Work out the finished part from the listing and answer in its coordinate system (mm). A direction names the side the tool comes from. Give positions to 0.01 mm unless a question says otherwise; leave off trailing zeros. Loops run counter-clockwise (first coordinate to the right, second up) from the corner with the lowest first, then second, coordinate; pieces in that order, holes last. Notation, with made-up numbers: M 18.25,34 L 22.25,34 A35 ccw 22.25,70 Z; hole C -39,-37 d10. An arc over 180 degrees is marked long. Use a Markdown table: item, result.
```python
from build123d import *

# Parameters (mm, degrees)
SKETCH1_W                 = 188.214
SKETCH1_H                 = 78.74
BOSS_EXTRUDE1_DEPTH       = 0.508
SKETCH1_3_W               = 188.214
SKETCH1_3_H               = 8.255
SKETCH1_3_H_2             = 78.74
SKETCH1_3_W_2             = 183.134
SKETCH1_3_H_3             = 73.66
BOSS_EXTRUDE2_DEPTH       = 27
BOSS_EXTRUDE3_START       = 21.59
BOSS_EXTRUDE3_DEPTH       = 32.5
SKETCH1_4_W               = 188.214
SKETCH1_4_H               = 8.255
BOSS_EXTRUDE4_DEPTH       = 0.508
F_4_40_TAPPED_HOLE2_D     = 2.2606
F_4_40_TAPPED_HOLE2_DEPTH = 7.62
F_4_40_TAPPED_HOLE2_TIP   = 0.679152758
SKETCH11_W                = 114.554
SKETCH11_H                = 8.255
SKETCH11_W_2              = 26.67
CUT_EXTRUDE1_DEPTH        = 28.508


with BuildPart() as part:
    # Sketch1 → Boss-Extrude1 (new body)
    with BuildSketch(Plane(origin=(0, 0, 0), x_dir=(1, 0, 0), z_dir=(0, 1, 0))):
        with Locations((94.107, -39.37)):
            Rectangle(SKETCH1_W, SKETCH1_H)
    extrude(amount=-BOSS_EXTRUDE1_DEPTH)

    # Sketch1<3> → Boss-Extrude2 (add)
    with BuildSketch(Plane(origin=(0, 0, 0), x_dir=(1, 0, 0), z_dir=(0, 1, 0))):
        with Locations((94.107, 4.1275)):
            Rectangle(SKETCH1_3_W, SKETCH1_3_H)
        with Locations((94.107, -82.8675)):
            Rectangle(SKETCH1_3_W, SKETCH1_3_H)
        with Locations((94.107, -39.37)):
            Rectangle(SKETCH1_3_W, SKETCH1_3_H_2)
        with Locations((94.107, -39.37)):
            Rectangle(SKETCH1_3_W_2, SKETCH1_3_H_3, mode=Mode.SUBTRACT)
    extrude(amount=BOSS_EXTRUDE2_DEPTH)

    # Sketch5 → Boss-Extrude3 (add)
    with BuildSketch(Plane.XY.offset(2.54).offset(BOSS_EXTRUDE3_START)):
        with BuildLine():
            Line((29.54, 7), (27.54, 7))
            ThreePointArc((27.54, 7), (23.600043647, 1.985651932), (17.54, 0))
            Line((17.54, 0), (39.54, 0))
            ThreePointArc((39.54, 0), (33.479956353, 1.985651932), (29.54, 7))
        make_face()
        with BuildLine():
            Line((55.4988, 7), (53.4988, 7))
            ThreePointArc((53.4988, 7), (49.558843647, 1.985651932), (43.4988, 0))
            Line((43.4988, 0), (65.4988, 0))
            ThreePointArc((65.4988, 0), (59.438756353, 1.985651932), (55.4988, 7))
        make_face()
        with BuildLine():
            Line((81.4576, 7), (79.4576, 7))
            ThreePointArc((79.4576, 7), (75.517643647, 1.985651932), (69.4576, 0))
            Line((69.4576, 0), (91.4576, 0))
            ThreePointArc((91.4576, 0), (85.397556353, 1.985651932), (81.4576, 7))
        make_face()
        with BuildLine():
            Line((107.4164, 7), (105.4164, 7))
            ThreePointArc((105.4164, 7), (101.476443647, 1.985651932), (95.4164, 0))
            Line((95.4164, 0), (117.4164, 0))
            ThreePointArc((117.4164, 0), (111.356356353, 1.985651932), (107.4164, 7))
        make_face()
        with BuildLine():
            Line((133.3752, 7), (131.3752, 7))
            ThreePointArc((131.3752, 7), (127.435243647, 1.985651932), (121.3752, 0))
            Line((121.3752, 0), (143.3752, 0))
            ThreePointArc((143.3752, 0), (137.315156353, 1.985651932), (133.3752, 7))
        make_face()
        with BuildLine():
            Line((159.334, 7), (157.334, 7))
            ThreePointArc((157.334, 7), (153.394043647, 1.985651932), (147.334, 0))
            Line((147.334, 0), (169.334, 0))
            ThreePointArc((169.334, 0), (163.273956353, 1.985651932), (159.334, 7))
        make_face()
    extrude(amount=BOSS_EXTRUDE3_DEPTH)

    # Sketch1<4> → Boss-Extrude4 (add)
    with BuildSketch(Plane(origin=(0, 0, 0), x_dir=(1, 0, 0), z_dir=(0, 1, 0))):
        with Locations((94.107, 4.1275)):
            Rectangle(SKETCH1_4_W, SKETCH1_4_H)
        with Locations((94.107, -82.8675)):
            Rectangle(SKETCH1_4_W, SKETCH1_4_H)
    extrude(amount=-BOSS_EXTRUDE4_DEPTH)

    # #4-40 Tapped Hole2
    with Locations(Plane(origin=(0, 27, 0), x_dir=(-1, 0, 0), z_dir=(0, 1, 0))):
        with Locations((-31.75, 0), (-156.464, 0), (-31.75, 78.74), (-156.464, 78.74)):
            Hole(F_4_40_TAPPED_HOLE2_D / 2, depth=F_4_40_TAPPED_HOLE2_DEPTH)
            with Locations((0, 0, -(F_4_40_TAPPED_HOLE2_DEPTH + F_4_40_TAPPED_HOLE2_TIP / 2))):  # 118° drill point
                Cone(0, F_4_40_TAPPED_HOLE2_D / 2, F_4_40_TAPPED_HOLE2_TIP, mode=Mode.SUBTRACT)

    # Sketch11 → Cut-Extrude1 (cut, through all)
    with BuildSketch(Plane(origin=(0, 27, 0), x_dir=(1, 0, 0), z_dir=(0, 1, 0))):
        with Locations((94.107, 4.1275)):
            Rectangle(SKETCH11_W, SKETCH11_H)
        with Locations((94.107, -82.8675)):
            Rectangle(SKETCH11_W, SKETCH11_H)
        with Locations((13.335, 4.1275)):
            Rectangle(SKETCH11_W_2, SKETCH11_H)
        with Locations((174.879, 4.1275)):
            Rectangle(SKETCH11_W_2, SKETCH11_H)
        with Locations((174.879, -82.8675)):
            Rectangle(SKETCH11_W_2, SKETCH11_H)
        with Locations((13.335, -82.8675)):
            Rectangle(SKETCH11_W_2, SKETCH11_H)
    extrude(amount=-CUT_EXTRUDE1_DEPTH, mode=Mode.SUBTRACT)


solid = part.part
```
(1) A cutting plane is placed at A-A (y = 12.5). Write down the section's boundary in (x, z) (3 decimals), and give its area (3 significant figures).
Entries:
| item | result |
|---|---|
| outline | M 0,0 L 26.67,0 L 26.67,-8.255 L 36.83,-8.255 L 36.83,0 L 151.384,0 L 151.384,-8.255 L 161.544,-8.255 L 161.544,0 L 188.214,0 L 188.214,78.74 L 161.544,78.74 L 161.544,86.995 L 151.384,86.995 L 151.384,78.74 L 36.83,78.74 L 36.83,86.995 L 26.67,86.995 L 26.67,78.74 L 0,78.74 Z; hole M 2.54,2.54 L 185.674,2.54 L 185.674,76.2 L 2.54,76.2 Z |
| area | 1,670 mm² |
(2) Given P1, Ø0.6, axis at x = 106, z = 47.5, coming from the +Y side; P2, Ø8, axis at x = 71.5, y = 15, coming from the -Z side; P3, Ø3.5, axis at x = 102.5, y = 4.5, coming from the +Z side, each flat-ended and moving along its own axis, determine where each tip first touches the part or whether it passes through.
Entries:
| item | result |
|---|---|
| P1 | stops at y = 7 |
| P2 | stops at z = 0 |
| P3 | stops at z = 78.74 |
(3) A cutting plane is placed at C-C (x = 114.5). Write down the section's boundary in (y, z), and give its area (3 significant figures).
Entries:
| item | result |
|---|---|
| outline | M -0.51,0 L 27,0 L 27,2.54 L 0,2.54 L 0,24.13 L 0.46,24.13 L 0.46,56.63 L 0,56.63 L 0,76.2 L 27,76.2 L 27,78.74 L -0.51,78.74 Z |
| area | 192 mm² |
(4) A cutting plane is placed at D-D (z = 68.5). Write down the section's boundary in (x, y), and give its area (3 significant figures).
Entries:
| item | result |
|---|---|
| outline | M 0,-0.51 L 188.21,-0.51 L 188.21,27 L 185.67,27 L 185.67,0 L 2.54,0 L 2.54,27 L 0,27 Z |
| area | 233 mm² |
(5) The mould has two halves that part along Z. Classify faces 1 (the flat face through (132, 2, 24.13)), 2 (the flat face through (13, 13, 78.74)), 3 (the flat face through (151.384, 13, 83)): released by +Z, released by -Z, zero draft, split by the parting line, or undercut.
Entries:
| item | result |
|---|---|
| face 1 | undercut |
| face 2 | released by +Z |
| face 3 | zero draft |
(6) Which of the six approach directions +Z, -Z, +X, -X, +Y, -Y give full straight-line access (tool end or side, diameter ignored) to faces 4 (the cylindrical face through (101.55, 2.04, 40.15)), 5 (the flat face through (36.83, 13, 83)), 6 (the flat face through (32, 13, 86.995)), 7 (the flat face through (0, 13, 40)), 8 (the flat face through (175, 13, 78.74))?
Entries:
| item | result |
|---|---|
| face 4 | +Y |
| face 5 | +Z, +Y, -Y |
| face 6 | +Z, +X, -X, +Y, -Y |
| face 7 | +Z, -Z, -X, +Y, -Y |
| face 8 | +Z, +X, +Y, -Y |
(7) Consider probe 1 along Z at (x, y) = (78.5, 0.5); probe 2 along Z at (x, y) = (178, 2.5); probe 3 along X at (y, z) = (24.5, 61). Determine where each line is inside the solid, lowest interval first. Write a range as [from, to].
Entries:
| item | result |
|---|---|
| probe 1 | z = [0, 2.54], [24.13, 56.63], [76.2, 78.74] |
| probe 2 | z = [0, 2.54], [76.2, 78.74] |
| probe 3 | x = [0, 2.54], [185.67, 188.21] |
